```python
from build123d import *

# Parameters (mm, degrees)
F0_W          = 20
F0_H          = 20
F1_DEPTH      = 50
F2_W          = 10
F2_H          = 3
F3_DEPTH      = 25
F3_DEPTH_BACK = 25
F4_R          = 4.99999
F5_R          = 2.5
F6_DEPTH      = 10
F7_R          = 4.99999
F8_W          = 3
F8_H          = 10
F9_DEPTH      = 25
F10_R         = 4.99999
F12_DEPTH     = 25
F13_R         = 4.99999
F11_R         = 2.5
F14_DEPTH     = 10


# Not quite as in the source:
# - a fillet or chamfer is up to 0.001 mm smaller than in the source, because OpenCascade refuses the exact size
# - a feature names something its author has since deleted; it is built from what else it names


with BuildPart() as f1:
    # F0 (on Front) → F1 (new body, symmetric)
    with BuildSketch(Plane.XZ):
        Rectangle(F0_W, F0_H)
    extrude(amount=F1_DEPTH, both=True)

    # F2 (on Right) → F3 (join, two sides)
    with BuildSketch(Plane.YZ) as f3_sk:
        with Locations((-40, 8.5)):
            Rectangle(F2_W, F2_H)
        with Locations((-40, -8.5)):
            Rectangle(F2_W, F2_H)
        with Locations((40, -8.5)):
            Rectangle(F2_W, F2_H)
        with Locations((40, 8.5)):
            Rectangle(F2_W, F2_H)
        with Locations((0, 8.5)):
            Rectangle(F2_W, F2_H)
        with Locations((0, -8.5)):
            Rectangle(F2_W, F2_H)
    extrude(amount=F3_DEPTH)
    extrude(f3_sk.sketch, amount=-F3_DEPTH_BACK)

    # F4 (radius 5 in the source; OpenCascade refuses exactly that, so slightly less here)
    f4_edges = [f1.edges().sort_by_distance(p)[0] for p in [
        (25, -45, 8.5),
        (25, -35, 8.5),
        (25, -45, -8.5),
        (25, -35, -8.5),
        (25, -5, 8.5),
        (25, 5, 8.5),
        (25, -5, -8.5),
        (25, 5, -8.5),
        (25, 35, 8.5),
        (25, 45, 8.5),
        (25, 35, -8.5),
        (25, 45, -8.5),
    ]]
    fillet(f4_edges, radius=F4_R)

    # F5 (on Top) → F6 (cut, symmetric)
    with BuildSketch(Plane.XY):
        with Locations((20, -40)):
            Circle(F5_R)
        with Locations((20, 40)):
            Circle(F5_R)
        with Locations((20, 0)):
            Circle(F5_R)
        with Locations((-20, -40)):
            Circle(F5_R)
        with Locations((-20, 0)):
            Circle(F5_R)
        with Locations((-20, 40)):
            Circle(F5_R)
    extrude(amount=F6_DEPTH, both=True, mode=Mode.SUBTRACT)

    # F7 (radius 5 in the source; OpenCascade refuses exactly that, so slightly less here)
    f7_edges = [f1.edges().sort_by_distance(p)[0] for p in [
        (-25, -45, -8.5),
        (-25, -35, -8.5),
        (-25, -45, 8.5),
        (-25, -35, 8.5),
        (-25, -5, -8.5),
        (-25, 5, -8.5),
        (-25, -5, 8.5),
        (-25, 5, 8.5),
        (-25, 35, -8.5),
        (-25, 45, -8.5),
        (-25, 35, 8.5),
        (-25, 45, 8.5),
    ]]
    fillet(f7_edges, radius=F7_R)

    # F8 (on Top) → F9 (join)
    with BuildSketch(Plane.XY):
        with Locations((8.5, 0)):
            Rectangle(F8_W, F8_H)
        with Locations((-8.5, 0)):
            Rectangle(F8_W, F8_H)
        with Locations((8.5, 40)):
            Rectangle(F8_W, F8_H)
        with Locations((-8.5, 40)):
            Rectangle(F8_W, F8_H)
        with Locations((-8.5, -40)):
            Rectangle(F8_W, F8_H)
        with Locations((8.5, -40)):
            Rectangle(F8_W, F8_H)
    extrude(amount=F9_DEPTH)

    # F10 (radius 5 in the source; OpenCascade refuses exactly that, so slightly less here)
    f10_edges = [f1.edges().sort_by_distance(p)[0] for p in [
        (8.5, -5, 25),
        (8.5, 5, 25),
        (-8.5, -5, 25),
        (-8.5, 5, 25),
    ]]
    fillet(f10_edges, radius=F10_R)

    # F8 (on Top) → F12 (join)
    with BuildSketch(Plane.XY):
        with Locations((8.5, 0)):
            Rectangle(F8_W, F8_H)
        with Locations((-8.5, 0)):
            Rectangle(F8_W, F8_H)
        with Locations((8.5, 40)):
            Rectangle(F8_W, F8_H)
        with Locations((-8.5, 40)):
            Rectangle(F8_W, F8_H)
        with Locations((-8.5, -40)):
            Rectangle(F8_W, F8_H)
        with Locations((8.5, -40)):
            Rectangle(F8_W, F8_H)
    extrude(amount=F12_DEPTH)

    # F13 (radius 5 in the source; OpenCascade refuses exactly that, so slightly less here)
    f13_edges = [f1.edges().sort_by_distance(p)[0] for p in [
        (8.5, 45, 25),
        (-8.5, 45, 25),
        (-8.5, 35, 25),
        (8.5, 35, 25),
        (8.5, 5, 25),
        (8.5, -5, 25),
        (-8.5, 5, 25),
        (-8.5, -5, 25),
        (8.5, -35, 25),
        (8.5, -45, 25),
        (-8.5, -35, 25),
        (-8.5, -45, 25),
    ]]
    fillet(f13_edges, radius=F13_R)

    # F11 (on Right) → F14 (cut, symmetric)
    with BuildSketch(Plane.YZ):
        with Locations((-40, 20)):
            Circle(F11_R)
        with Locations((40, 20)):
            Circle(F11_R)
        with Locations((0, 20)):
            Circle(F11_R)
    extrude(amount=F14_DEPTH, both=True, mode=Mode.SUBTRACT)


solid = f1.part
```
Verification items for the finished model (mm, model axes). A direction names the side the tool comes from. Give positions to 0.01 mm unless a question says otherwise; leave off trailing zeros. Loops run counter-clockwise (first coordinate to the right, second up) from the corner with the lowest first, then second, coordinate; pieces in that order, holes last.
1. Section check A-A, the plane z = 16. Enter the section's corners in (x, y), then the cut area to 3 significant figures.
2. Set-up check for faces 4 (the flat face through (-15, -45, -9)), 5 (the flat face through (16, 40, 10)), 6 (the flat face through (15, -45, -9)), 7 (the flat face through (-10, 40, 16)), 8 (the flat face through (-9, 35, 15)): record each of +Z, -Z, +X, -X, +Y, -Y from which the full face is reachable in a straight line by a thin tool's end or side.
3. Section check B-B, the plane x = 9. Count the separate pieces of the cut face and the enclosed holes in it, then the cut area to 3 significant figures.
4. Mould release check, pull along Z, two halves, no side actions. Record for faces 1 (the cylindrical face through (17.5, -39.9, -8.5)), 2 (the flat face through (-16, -40, 10)), 3 (the flat face through (16, 40, -7)): released by +Z, released by -Z, zero draft, split by the parting line, or undercut.
5. Section check D-D, the plane z = 3. Enter the section's corners in (x, y).
6. Go/stop test with flat-tipped pins: pin 1 Ø6 at (x, y) = (-8.5, 6) entering from +Z; pin 2 Ø12 at (x, z) = (-15.5, 13.5) entering from +Y; pin 3 Ø3.5 at (x, z) = (15.5, 8) entering from -Y. Record where each tip stops, or that it passes through.
7. Thickness scan on line 1 (Y direction, x = 14, z = 8); line 2 (Y direction, x = 20, z = -9); line 3 (Z direction, x = -8, y = 0). Record the ranges inside material, lowest first.
8. Section check C-C, the plane y = 43.5. Enter the section's corners in (x, z).
Geometry says:
1. outline: (-10, -45) - (-7, -45) - (-7, -35) - (-10, -35) - close; (-10, -5) - (-7, -5) - (-7, 5) - (-10, 5) - close; (-10, 35) - (-7, 35) - (-7, 45) - (-10, 45) - close; (7, -45) - (10, -45) - (10, -35) - (7, -35) - close; (7, -5) - (10, -5) - (10, 5) - (7, 5) - close; (7, 35) - (10, 35) - (10, 45) - (7, 45) - close
1. area: 180 mm2
2. face 4: +Z, -Z, -X, -Y
2. face 5: +Z, +X, +Y, -Y
2. face 6: +Z, -Z, +X, -Y
2. face 7: +Z, -X, +Y, -Y
2. face 8: +Z, +X, -X
3. separate pieces: 1
3. enclosed holes: 3
3. area: 2,360 mm2
4. face 1: zero draft
4. face 2: released by +Z
4. face 3: undercut
5. outline: (-10, -50) - (10, -50) - (10, 50) - (-10, 50) - close
6. pin 1: stops at z = 24
6. pin 2: stops at y = 45
6. pin 3: stops at y = -45
7. line 1: y = -45 to -35, -5 to 5, 35 to 45
7. line 2: y = -45 to -42.5, -37.5 to -35, -5 to -2.5, 2.5 to 5, 35 to 37.5, 42.5 to 45
7. line 3: z = -10 to 17.5, 22.5 to 25
8. outline: (-23.57, -10) - (23.57, -10) - (23.57, -7) - (10, -7) - (10, 7) - (23.57, 7) - (23.57, 10) - (10, 10) - (10, 23.57) - (7, 23.57) - (7, 10) - (-7, 10) - (-7, 23.57) - (-10, 23.57) - (-10, 10) - (-23.57, 10) - (-23.57, 7) - (-10, 7) - (-10, -7) - (-23.57, -7) - close
